Build history of the part. All positions in model axes, mm. A direction names the side the tool comes from. Round coordinates to 2 decimals unless told otherwise and drop trailing zeros. Write each loop counter-clockwise with the first axis right and the second up, starting at its lowest first coordinate (ties: lowest second). Pieces come first, ordered by that corner, then holes. Notation, with made-up numbers: M 77.5,6.5 L 115.5,6.5 A27 cw 115.5,33.5 Z; hole C 79,18.5 d10. An arc over 180 degrees is marked long. Write item = value, one per line.
from build123d import *

# Parameters (mm, degrees)
SALIENTE_EXTRUIR1_DEPTH    = 63.5
CORTAR_EXTRUIR1_DEPTH      = 57
CORTAR_EXTRUIR1_DEPTH_BACK = 42
CROQUIS6_R                 = 5
CORTAR_EXTRUIR2_REACH      = 89.824
CORTAR_EXTRUIR2_END_RADIUS = 5
CROQUIS7_R                 = 2


with BuildPart() as part:
    # Croquis1 → Saliente-Extruir1 (new, symmetric)
    with BuildSketch(Plane(origin=(0, 0, 0), x_dir=(0, 0, -1), z_dir=(1, 0, 0))):
        Polygon((-9.6, 25.4), (-25.4, 9.6), (-25.4, -25.4), (25.4, -25.4), (25.4, 25.4), align=None)
    extrude(amount=SALIENTE_EXTRUIR1_DEPTH, both=True)

    # Croquis5 → Taladro roscado 1/4 NPT2 (revolve, cut)
    with BuildSketch(Plane(origin=(-63.5, 0, 0), x_dir=(0, 0, 1), z_dir=(0, 1, 0))):
        Polygon((0, 0), (0, 23.342347279), (5.5626, 20), (5.5626, 10.02), (6.557975082, 10.02), (6.8579873, 0), align=None)
    revolve(axis=Axis((-69.85, 0, 0), (1, 0, 0)), mode=Mode.SUBTRACT)

    # Croquis6 → Cortar-Extruir1 (cut, two sides: drawn at the far end of the back side and taken through both)
    with BuildSketch(Plane(origin=(0, 0, 0), x_dir=(0, 0, -1), z_dir=(1, 0, 0)).offset(-CORTAR_EXTRUIR1_DEPTH_BACK)):
        Circle(CROQUIS6_R)
    extrude(amount=CORTAR_EXTRUIR1_DEPTH + CORTAR_EXTRUIR1_DEPTH_BACK, mode=Mode.SUBTRACT)

    # Cortar-Extruir2: up to this cylinder (the profile starts outside it)
    cortar_extruir2_end = Plane(origin=(0, 0, 0), z_dir=(-1, 0, 0)) * Cylinder(CORTAR_EXTRUIR2_END_RADIUS, 290.648, mode=Mode.PRIVATE)
    # Croquis7 → Cortar-Extruir2 (cut, up to the surface)
    with BuildSketch(Plane(origin=(0, 17.5, 17.5), x_dir=(1, 0, 0), z_dir=(0, 0.7071067811865479, 0.7071067811865472)), mode=Mode.PRIVATE) as cortar_extruir2_sk1:
        with Locations(Location((0, 0, 0), (0, 0, 270))):
            Circle(CROQUIS7_R)
    cortar_extruir2_tool1 = extrude(cortar_extruir2_sk1.sketch, amount=-CORTAR_EXTRUIR2_REACH, mode=Mode.PRIVATE) - cortar_extruir2_end
    add(cortar_extruir2_tool1.solids().sort_by_distance((0, 17.5, 17.5))[0], mode=Mode.SUBTRACT)
    # Croquis7 → Cortar-Extruir2 (cut, up to the surface)
    with BuildSketch(Plane(origin=(0, 17.5, 17.5), x_dir=(1, 0, 0), z_dir=(0, 0.7071067811865479, 0.7071067811865472)), mode=Mode.PRIVATE) as cortar_extruir2_sk2:
        with Locations(Location((25, 0, 0), (0, 0, 270))):
            Circle(CROQUIS7_R)
    cortar_extruir2_tool2 = extrude(cortar_extruir2_sk2.sketch, amount=-CORTAR_EXTRUIR2_REACH, mode=Mode.PRIVATE) - cortar_extruir2_end
    add(cortar_extruir2_tool2.solids().sort_by_distance((25, 17.5, 17.5))[0], mode=Mode.SUBTRACT)
    # Croquis7 → Cortar-Extruir2 (cut, up to the surface)
    with BuildSketch(Plane(origin=(0, 17.5, 17.5), x_dir=(1, 0, 0), z_dir=(0, 0.7071067811865479, 0.7071067811865472)), mode=Mode.PRIVATE) as cortar_extruir2_sk3:
        with Locations(Location((50, 0, 0), (0, 0, 270))):
            Circle(CROQUIS7_R)
    cortar_extruir2_tool3 = extrude(cortar_extruir2_sk3.sketch, amount=-CORTAR_EXTRUIR2_REACH, mode=Mode.PRIVATE) - cortar_extruir2_end
    add(cortar_extruir2_tool3.solids().sort_by_distance((50, 17.5, 17.5))[0], mode=Mode.SUBTRACT)
    # Croquis7 → Cortar-Extruir2 (cut, up to the surface)
    with BuildSketch(Plane(origin=(0, 17.5, 17.5), x_dir=(1, 0, 0), z_dir=(0, 0.7071067811865479, 0.7071067811865472)), mode=Mode.PRIVATE) as cortar_extruir2_sk4:
        with Locations(Location((-50, 0, 0), (0, 0, 270))):
            Circle(CROQUIS7_R)
    cortar_extruir2_tool4 = extrude(cortar_extruir2_sk4.sketch, amount=-CORTAR_EXTRUIR2_REACH, mode=Mode.PRIVATE) - cortar_extruir2_end
    add(cortar_extruir2_tool4.solids().sort_by_distance((-50, 17.5, 17.5))[0], mode=Mode.SUBTRACT)
    # Croquis7 → Cortar-Extruir2 (cut, up to the surface)
    with BuildSketch(Plane(origin=(0, 17.5, 17.5), x_dir=(1, 0, 0), z_dir=(0, 0.7071067811865479, 0.7071067811865472)), mode=Mode.PRIVATE) as cortar_extruir2_sk5:
        with Locations(Location((-25, 0, 0), (0, 0, 270))):
            Circle(CROQUIS7_R)
    cortar_extruir2_tool5 = extrude(cortar_extruir2_sk5.sketch, amount=-CORTAR_EXTRUIR2_REACH, mode=Mode.PRIVATE) - cortar_extruir2_end
    add(cortar_extruir2_tool5.solids().sort_by_distance((-25, 17.5, 17.5))[0], mode=Mode.SUBTRACT)


solid = part.part
1. Probe probe 1 along Y at (x, z) = (-46, 0); probe 2 along Y at (x, z) = (25, 0). List the from-to ranges inside material, lowest first.
Responses:
probe_1 = -25.4 to -5.56, 5.56 to 25.4
probe_2 = -25.4 to -5, 5 to 25.4
2. Tool access for faces 1 (the face through (-53.48, 5, 3)), 2 (the face through (6.807, -1.915, -4.619)), 3 (the face through (1, -25.4, 0)): list every direction of +Z, -Z, +X, -X, +Y, -Y with a clear straight run to the whole face (end or side of a thin tool).
Responses:
face_1 = -X
face_2 = none
face_3 = +Z, -Z, +X, -X, -Y
3. Band-saw the part on B-B (y = 0). List the corners of the cut face in (x, z).
Responses:
outline = M -63.5,-25.4 L 63.5,-25.4 L 63.5,25.4 L -63.5,25.4 L -63.5,6.86 L -53.48,6.56 L -53.48,5.56 L -43.5,5.56 L -42,3.07 L -42,5 L 57,5 L 57,-5 L -42,-5 L -42,-3.07 L -43.5,-5.56 L -53.48,-5.56 L -53.48,-6.56 L -63.5,-6.86 Z
4. Mould opens along Y. For faces 4 (the face through (-63.5, -5, -5)), 5 (the face through (1, 19, 16)), 6 (the face through (-42, -1, -3.3)) say: pulls with the +Y half, pulls with the -Y half, needs draft (parallel to the pull), parting line crosses it, or undercut.
Responses:
face_4 = needs draft
face_5 = pulls with the +Y half
face_6 = undercut
5. Band-saw the part on A-A (x = -3.5). List the corners of the cut face in (y, z), plus the area to 3 significant figures.
Responses:
outline = M -25.4,-25.4 L 25.4,-25.4 L 25.4,9.6 L 9.6,25.4 L -25.4,25.4 Z; hole C 0,0 d10
area = 2,380 mm²
6. Flat gauge pins, fed straight in: pin 1 (4 mm diameter, centred on y = 3, z = 1.5, fed in from -X); pin 2 (1.5 mm diameter, centred on x = 47.5, y = 17.5, fed in from +Z); pin 3 (11.5 mm diameter, centred on y = 0, z = 0, fed in from -X). Where does each tip first touch, or does it go through?
Responses:
pin_1 = -43.37
pin_2 = 18.25
pin_3 = -53.48
